Read the model definition and answer for the solid it produces. Units are mm, in the model's axes. A direction names the side the tool comes from. Round coordinates to 2 decimals unless told otherwise and drop trailing zeros. Write each loop counter-clockwise with the first axis right and the second up, starting at its lowest first coordinate (ties: lowest second). Pieces come first, ordered by that corner, then holes. Notation, with made-up numbers: (-22, 1) -> (7, 1) arc R36 ccw to (7, 40) -> close; hole circle Ø4 at (62, 10). An arc over 180 degrees is marked (long way). Return JSON: item names as keys, results as strings.
from build123d import *

# Parameters (mm, degrees)
SKETCH11_W          = 36
SKETCH11_H          = 12
BOSS_EXTRUDE3_DEPTH = 1.2
EXTRUDE_THIN2_START = 36
EXTRUDE_THIN2_DEPTH = 10


with BuildPart() as part:
    # Sketch11 → Boss-Extrude3 (new body)
    with BuildSketch(Plane.XY):
        with Locations((18, 6)):
            Rectangle(SKETCH11_W, SKETCH11_H)
    extrude(amount=BOSS_EXTRUDE3_DEPTH)

    # Sketch2 → Extrude-Thin2 (add)
    with BuildSketch(Plane(origin=(0, 0, 0), x_dir=(0, 0, -1), z_dir=(1, 0, 0)).offset(EXTRUDE_THIN2_START)):
        with BuildLine():
            ThreePointArc((0, 0), (2.668251438, 3.477332975), (6.717691454, 1.8))
            Line((6.717691454, 1.8), (7.756921938, 2.4))
            ThreePointArc((7.756921938, 2.4), (2.357668584, 4.636443966), (-1.2, 0))
            Line((-1.2, 0), (0, 0))
        make_face()
    extrude(amount=-EXTRUDE_THIN2_DEPTH)

    # Mirror1: part across plane


with BuildPart() as part_1:
    add(part.part)
    add(part.part.mirror(Plane.ZX))


solid = part_1.part
Item 1: Flat-ended cylindrical pins translate along their axes: pin 1 (1.4 mm diameter, centred on y = -1.5, z = -5, fed in from -X); pin 2 (4 mm diameter, centred on y = 2.5, z = -3, fed in from -X). Find the tip coordinate at first contact, or state that the pin passes through.
Worked answers:
{"pin 1": "passes through", "pin 2": "stops at x = 26"}
Item 2: Section D-D (z = -2.25) is taken. Give the vertices of the cut face in (x, y), then the cut area to 3 significant figures.
Worked answers:
{"outline": "(26, -4.61) -> (36, -4.61) -> (36, -3.34) -> (26, -3.34) -> close; (26, 3.34) -> (36, 3.34) -> (36, 4.61) -> (26, 4.61) -> close", "area": "25.4 mm2"}
Item 3: A tool of negligible diameter and unlimited length cuts with its end or side. For faces 4 (the flat face through (31.07, -2.096, -7.23)), 5 (the flat face through (18, 12, 1)), 6 (the flat face through (26, 4, -4)), from which of +Z, -Z, +X, -X, +Y, -Y can it reach the whole face along a straight path? Write none if from no direction.
Worked answers:
{"face 4": "-Z, +X, -X", "face 5": "+Z, -Z, +X, -X, +Y", "face 6": "-Z, -X, +Y, -Y"}
Item 4: For a pull along Z with two mould halves and no side action, classify faces 1 (the cylindrical face through (31.07, 4.77, -4.14)), 2 (the flat face through (31.07, 2.096, -7.23)), 3 (the flat face through (0, 0, 1)) as released by +Z, released by -Z, zero draft, split by the parting line, or undercut.
Worked answers:
{"face 1": "undercut", "face 2": "released by -Z", "face 3": "zero draft"}
Item 5: Section B-B (y = 6.25) is taken. Give the vertices of the cut face in (x, z), then the cut area to 3 significant figures.
Worked answers:
{"outline": "(0, 0) -> (36, 0) -> (36, 1.2) -> (0, 1.2) -> close", "area": "43.2 mm2"}
Item 6: Section C-C (x = 32.5) is taken. Give the vertices of the cut face in (y, z).
Worked answers:
{"outline": "(-12, 0) -> (-3.17, 0) arc R4.8 ccw to (-2.4, -7.76) -> (-1.8, -6.72) arc R3.6 cw (long way) to (1.8, -6.72) -> (2.4, -7.76) arc R4.8 ccw to (3.17, 0) -> (12, 0) -> (12, 1.2) -> (-12, 1.2) -> close"}
Item 7: Section A-A (z = -4) is taken. Give the vertices of the cut face in (x, y).
Worked answers:
{"outline": "(26, -4.78) -> (36, -4.78) -> (36, -3.58) -> (26, -3.58) -> close; (26, 3.58) -> (36, 3.58) -> (36, 4.78) -> (26, 4.78) -> close"}
Item 8: Straight lines are drawn through the part: L1, parallel to Z at x = 13.5, y = 1.5; L2, parallel to Z at x = 28.5, y = 4.25; L3, parallel to Y at x = 27, z = -3. For each, find the intervals that lie inside material, in ascending order. Write a range as [from, to].
Worked answers:
{"L1": "z = [0, 1.2]", "L2": "z = [-5.83, -1.37], [0, 1.2]", "L3": "y = [-4.76, -3.55], [3.55, 4.76]"}
